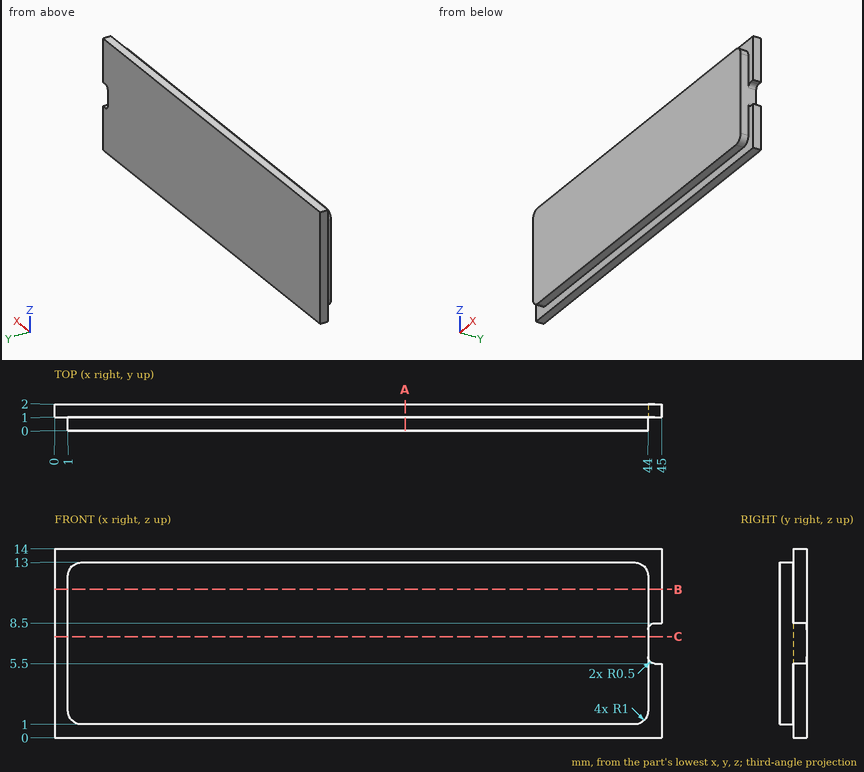
For this review, use the dimensioned drawing (mm, ordinates from the lowest corner) and the shaded views. Round coordinates to 2 decimals unless told otherwise and drop trailing zeros. Order: outer loops, then holes, each group sorted by start corner. A loop starts at its lowest first (then second) coordinate and runs counter-clockwise, first axis right, second up. Notation, with made-up numbers: (15, 10.5) -> (39, 10.5) arc R16 cw to (39, 33.5) -> close; hole circle Ø2 at (14.25, 7). An arc over 180 degrees is marked (long way). Write item = value, one per line. Start each with the question number.
Item 1: Consider section A-A on x = 26. Write out the cut boundary in (y, z), plus the area to 3 significant figures.
Item 2: Consider section C-C on z = 7.5. Write out the cut boundary in (x, y).
Item 3: For line 1 along Z through (x, y) = (18, 0.9); line 2 along X through (y, z) = (0.9, 11.5); line 3 along Y through (x, z) = (5, 0.5), list the stretches that pass through material, from the lowest coordinate up.
Item 4: Clearance check with a flat-ended pin moving along its axis: pin 1 Ø0.8 at (x, y) = (29.5, 0.5) entering from -Z. State where the tip first meets the part, or that it passes through.
Item 5: Consider section B-B on z = 11. Write out the cut boundary in (x, y).
Conclusion:
q1.outline = (0, 1) -> (1, 1) -> (1, 0) -> (2, 0) -> (2, 14) -> (1, 14) -> (1, 13) -> (0, 13) -> close
q1.area = 26.0 mm2
q2.outline = (0, 1) -> (1, 1) -> (1, 0) -> (44, 0) -> (44, 2) -> (0, 2) -> close
q3.line_1 = 1 to 13
q3.line_2 = 1 to 44
q3.line_3 = 1 to 2
q4.pin_1 = 1
q5.outline = (0, 1) -> (1, 1) -> (1, 0) -> (44, 0) -> (44, 1) -> (45, 1) -> (45, 2) -> (0, 2) -> close
